```python
from build123d import *

# Parameters (mm, degrees)
SKETCH_W   = 50
SKETCH_H   = 50
SKETCH_W_2 = 44
SKETCH_H_2 = 44
PAD_DEPTH  = 100
FILLET_R   = 1


with BuildPart() as part:
    # Sketch → Pad (new body)
    with BuildSketch(Plane.XY):
        with Locations((25, 25)):
            Rectangle(SKETCH_W, SKETCH_H)
        with Locations((25, 25)):
            Rectangle(SKETCH_W_2, SKETCH_H_2, mode=Mode.SUBTRACT)
    extrude(amount=PAD_DEPTH)

    # Fillet
    fillet_edges = [part.edges().sort_by_distance(p)[0] for p in [
        (0, 50, 50),
        (50, 50, 50),
        (50, 0, 50),
        (0, 0, 50),
    ]]
    fillet(fillet_edges, radius=FILLET_R)


solid = part.part
```
Here's how the part is built. I have some questions about the finished solid (model axes, mm). A direction names the side the tool comes from. Coordinates: 2 decimals unless noted, no trailing zeros. Order: outer loops, then holes, each group sorted by start corner. A loop starts at its lowest first (then second) coordinate and runs counter-clockwise, first axis right, second up.
1) We'd pull the mould along Y, two halves only. Please class faces 1 (the face through (3, 25, 49)), 2 (the face through (25, 50, 49)), 3 (the face through (2.7, 25.1, 0)): +Y half, -Y half, draft (parallel to the pull), parting line (faces both ways), or undercut.
2) Imagine slicing it at A-A on x = 5. List the corners of the cut face in (y, z) for me, and give its area (3 significant figures).
3) I need wall thicknesses on line 1 (Y direction, x = 17.5, z = 93.5). Which ranges of the line are inside material? Lowest first, please.
4) Which directions (+Z, -Z, +X, -X, +Y, -Y) give clear straight access to the entire face, cutting with the end or side of a thin tool? Please do faces 4 (the face through (2.7, 25.1, 100)), 5 (the face through (25, 47, 49)).
5) Imagine slicing it at C-C on z = 89.5. List the corners of the cut face in (x, y) for me, and give its area (3 significant figures).
Response values:
1. face 1: undercut
1. face 2: +Y half
1. face 3: draft
2. outline: (0, 0) - (3, 0) - (3, 100) - (0, 100) - close; (47, 0) - (50, 0) - (50, 100) - (47, 100) - close
2. area: 600 mm2
3. line 1: y = 0 to 3, 47 to 50
4. face 4: +Z, +X, -X, +Y, -Y
4. face 5: +Z, -Z
5. outline: (0, 1) arc R1 ccw to (1, 0) - (49, 0) arc R1 ccw to (50, 1) - (50, 49) arc R1 ccw to (49, 50) - (1, 50) arc R1 ccw to (0, 49) - close; hole (3, 3) - (47, 3) - (47, 47) - (3, 47) - close
5. area: 563 mm2
